Model file for the job. Use its own axes, mm. A direction names the side the tool comes from. Coordinates: 2 decimals unless noted, no trailing zeros. Order: outer loops, then holes, each group sorted by start corner. A loop starts at its lowest first (then second) coordinate and runs counter-clockwise, first axis right, second up.
from build123d import *

# Parameters (mm, degrees)
F0_R        = 2.7305
F1_DEPTH    = 25.019
F2_R        = 2.54
F3_R        = 7.874
F4_R        = 5.08
F5_T1_DEPTH = 50.419


# Not quite as in the source:
# - a fillet or chamfer that OpenCascade refuses, or shapes differently, is made with other operations: its cross-section is extruded or revolved along the edge and cut away or added


with BuildPart() as f1:
    # F0 (on Front) → F1 (new body)
    with BuildSketch(Plane.XZ):
        Polygon((-6.7945, 10.795), (-21.9964, 10.795), (-21.9964, -2.159), (-16.3195, -2.159), (-16.3195, -10.795), (0, -10.795), (16.3195, -10.795), (16.3195, -2.159), (21.9964, -2.159), (21.9964, 10.795), (6.7945, 10.795), (6.7945, -2.159), (0, -2.159), (-6.7945, -2.159), align=None)
        with Locations((-14.1859, 2.6289)):
            Circle(F0_R, mode=Mode.SUBTRACT)
        with Locations((14.1859, 2.6289)):
            Circle(F0_R, mode=Mode.SUBTRACT)
    extrude(amount=F1_DEPTH)

    # F2
    f2_edges = [f1.edges().sort_by_distance(p)[0] for p in [
        (-6.7945, -12.5095, 10.795),
        (-6.7945, -12.5095, -2.159),
        (6.7945, -12.5095, -2.159),
        (6.7945, -12.5095, 10.795),
    ]]
    fillet(f2_edges, radius=F2_R)

    # F3
    f3_edges = [f1.edges().sort_by_distance(p)[0] for p in [
        (-21.9964, -12.5095, 10.795),
        (21.9964, -12.5095, 10.795),
    ]]
    fillet(f3_edges, radius=F3_R)

    # F4
    f4_edges = [f1.edges().sort_by_distance(p)[0] for p in [
        (-16.3195, -12.5095, -2.159),
        (16.3195, -12.5095, -2.159),
    ]]
    fillet(f4_edges, radius=F4_R)

    # F5: fillet of radius 7.874 on 2 edges, made by hand

    # F5_s2 → F5_t1 (cut)
    with BuildSketch(Plane.XZ.offset(-12.7)):
        with BuildLine():
            ThreePointArc((-18.5538606902, -3.0308249896), (-20.9591016403, -0.4505219212), (-21.9964, 2.921))
            Line((-21.9964, 2.921), (-22.781728024, 2.8639153723))
            ThreePointArc((-22.781728024, 2.8639153723), (-22.7838, 0.381), (-22.7838, -2.159))
            Line((-22.7838, -2.159), (-21.9964, -2.9464))
            ThreePointArc((-21.9964, -2.9464), (-21.3995, -2.9464), (-18.9949347832, -3.6830921162))
            Line((-18.9949347832, -3.6830921162), (-18.5538606902, -3.0308249896))
        make_face()
        with BuildLine():
            ThreePointArc((18.5538606902, -3.0308249896), (20.9591016403, -0.4505219212), (21.9964, 2.921))
            Line((21.9964, 2.921), (22.781728024, 2.8639153723))
            ThreePointArc((22.781728024, 2.8639153723), (22.7838, 0.381), (22.7838, -2.159))
            Line((22.7838, -2.159), (21.9964, -2.9464))
            ThreePointArc((21.9964, -2.9464), (21.3995, -2.9464), (18.9949347832, -3.6830921162))
            Line((18.9949347832, -3.6830921162), (18.5538606902, -3.0308249896))
        make_face()
    extrude(amount=F5_T1_DEPTH, mode=Mode.SUBTRACT)


solid = f1.part
Q1. Cut at D-D, the plane z = -9.5. List the corners of the cut face in (x, y).
Established:
outline: (-16.32, -25.02) - (16.32, -25.02) - (16.32, 0) - (-16.32, 0) - close
Q2. Cut at B-B, the plane z = 3.5. List the corners of the cut face in (x, y), plus the area to 3 significant figures.
Established:
outline: (-21.98, -25.02) - (-16.77, -25.02) - (-16.77, 0) - (-21.98, 0) - close; (-11.6, -25.02) - (-6.79, -25.02) - (-6.79, 0) - (-11.6, 0) - close; (6.79, -25.02) - (11.6, -25.02) - (11.6, 0) - (6.79, 0) - close; (16.77, -25.02) - (21.98, -25.02) - (21.98, 0) - (16.77, 0) - close
area: 501 mm2
Q3. Which spindle directions (+Z, -Z, +X, -X, +Y, -Y) get a long thin tool onto all of the face, cutting with end or side? Do faces 1 (the face through (6.031, -12.685, -1.435)), 2 (the face through (-19.63, -12.68, 8.55)), 3 (the face through (16.32, -12, -9)), 4 (the face through (-16.32, -12, -9)). Say none if no direction does.
Established:
face 1: +Z, +Y, -Y
face 2: +Z, -X, +Y, -Y
face 3: -Z, +X, +Y, -Y
face 4: -Z, -X, +Y, -Y
Q4. Probe line 1 (X direction, y = -21.5, z = 1.25); line 2 (X direction, y = -1.75, z = 1); line 3 (Z direction, x = -1, y = -10) (3 decimals). List the from-to ranges inside material, lowest first.
Established:
line 1: x = -21.69 to -16.54, -11.83 to -6.79, 6.79 to 11.83, 16.54 to 21.69
line 2: x = -21.61 to -16.38, -11.99 to -6.79, 6.79 to 11.99, 16.38 to 21.61
line 3: z = -10.795 to -2.159
Q5. Cut at C-C, the plane x = -1. List the corners of the cut face in (y, z) (3 decimals).
Established:
outline: (-25.019, -10.795) - (0, -10.795) - (0, -2.159) - (-25.019, -2.159) - close
Q6. Cut at A-A, the plane y = -14.5. List the corners of the cut face in (x, z) (1 decimal), plus the area to 3 significant figures.
Established:
outline: (-22, 2.9) arc R7.9 ccw to (-18.6, -3) arc R5.1 cw to (-16.3, -7.2) - (-16.3, -10.8) - (16.3, -10.8) - (16.3, -7.2) arc R5.1 cw to (18.6, -3) arc R7.9 ccw to (22, 2.9) arc R7.9 ccw to (14.1, 10.8) - (9.3, 10.8) arc R2.5 ccw to (6.8, 8.3) - (6.8, 0.4) arc R2.5 cw to (4.3, -2.2) - (-4.3, -2.2) arc R2.5 cw to (-6.8, 0.4) - (-6.8, 8.3) arc R2.5 ccw to (-9.3, 10.8) - (-14.1, 10.8) arc R7.9 ccw to start; hole circle Ø5.5 at (-14.2, 2.6); hole circle Ø5.5 at (14.2, 2.6)
area: 605 mm2
Q7. Mould opens along Z. For faces 5 (the face through (-20.934, -12.334, -0.494)), 6 (the face through (12.019, -12.334, 0.967)), 7 (the face through (0, 0, -5)) say: pulls with the +Z half, pulls with the -Z half, needs draft (parallel to the pull), parting line crosses it, or undercut.
Established:
face 5: pulls with the -Z half
face 6: undercut
face 7: needs draft
Q8. Drop flat-ended pins along their axis: P1, Ø10, axis at x = 6, z = -3.5, coming from the +Y side; P2, Ø1.5, axis at y = -7.5, z = -6.5, coming from the -X side; P3, Ø3, axis at y = -8.5, z = -10, coming from the +X side; P4, Ø8, axis at y = -15.5, z = -6, coming from the +X side. Give the stop position or say it passes through.
Established:
P1: stops at y = 0
P2: stops at x = -16.54
P3: stops at x = 16.32
P4: stops at x = 19.79
